Design review of the part built by this model. Coordinates are the model's own, in mm. Face numbers are marked on the shaded views. A direction names the side the tool comes from. Give positions to 0.01 mm unless a question says otherwise; leave off trailing zeros. Loops run counter-clockwise (first coordinate to the right, second up) from the corner with the lowest first, then second, coordinate; pieces in that order, holes last.
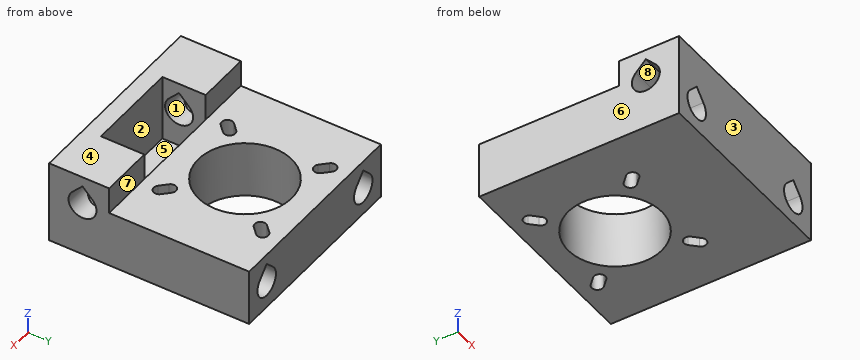
Solid Edge part; units mm, degrees
sketch "Sketch1" plane through (0, 0, 0) normal (0, 0, 1) x (1, 0, 0)
  circle A0 centre (-15.5, 15.5) radius 1.7
  circle A1 centre (15.5, 15.5) radius 1.7
  circle A2 centre (15.5, -15.5) radius 1.7
  circle A3 centre (-15.5, -15.5) radius 1.7
  line L0 (-30, -21) -> (30, -21)
  line L1 (30, -21) -> (30, 21)
  line L2 (30, 21) -> (-30, 21)
  line L3 (-30, 21) -> (-30, -21)
  circle A4 centre (0, 0) radius 14
  dimension "D1" = 30
  dimension "D2" = 30
extrude "Protrusion1" add sketch "Sketch1" along normal blind 17
sketch "Sketch2" plane through (30, 0, 8.5) normal (1, 0, 0) x (0, 1, 0)
  line L0 (-21, -8.5) -> (-39, -8.5)
  line L1 (-39, -8.5) -> (-39, 16.5)
  line L2 (-39, 16.5) -> (-21, 16.5)
  line L3 (-21, 16.5) -> (-21, -8.5)
  dimension "D1" = 21
  dimension "D2" = 39
extrude "Protrusion2" add sketch "Sketch2" against normal up to vertex (60 mm away)
sketch "Sketch3" plane through (0, 21, 8.5) normal (0, 1, 0) x (-1, 0, 0)
  line L0 (-22, 5.5461) -> (-25.0212, 2.4176)
  line L1 (-18.9788, 2.4176) -> (-22, 5.5461)
  arc A0 (-25.0212, 2.4176) -> (-18.9788, 2.4176) centre (-22, -0.5) ccw
  line L2 (22, 5.5461) -> (18.9788, 2.4176)
  line L3 (25.0212, 2.4176) -> (22, 5.5461)
  arc A1 (18.9788, 2.4176) -> (25.0212, 2.4176) centre (22, -0.5) ccw
  dimension "D1" = 22
extrude "Cutout1" cut sketch "Sketch3" against normal through all
sketch "Sketch4" plane through (30, -8, 12.5) normal (1, 0, 0) x (0, 1, 0)
  line L0 (-17.9788, 6.4176) -> (-21, 9.5461)
  line L1 (-21, 9.5461) -> (-24.0212, 6.4176)
  arc A0 (-24.0212, 6.4176) -> (-17.9788, 6.4176) centre (-21, 3.5) ccw
extrude "Cutout2" cut sketch "Sketch4" against normal through all
sketch "Sketch5" plane through (0, -30, 25) normal (0, 0, 1) x (0, -1, 0)
  line L0 (-9, -14) -> (4, -14)
  line L1 (4, -14) -> (4, 14)
  line L2 (4, 14) -> (-9, 14)
  line L3 (-9, 14) -> (-9, -14)
extrude "ExtrudedCutout_3" cut sketch "Sketch5" against normal blind 20
sketch "Sketch6" plane through (0, -9, 0) normal (0, 0, -1) x (0, 1, 0)
  line L0 (23.2979, 16.7021) -> (21.2958, 14.7)
  arc A0 (21.2958, 14.7) -> (23.7021, 12.2979) centre (22.499, 13.499) ccw
  line L1 (23.7021, 12.2979) -> (25.7021, 14.2979)
  line L2 (23.2979, 16.7021) -> (25.7021, 14.2979)
  line L3 (25.7021, -14.2979) -> (23.7, -12.2958)
  arc A1 (23.7, -12.2958) -> (21.2979, -14.7021) centre (22.499, -13.499) ccw
  line L4 (21.2979, -14.7021) -> (23.2979, -16.7021)
  arc A2 (25.7021, -14.2979) -> (23.2979, -16.7021) centre (24.5, -15.5) ccw
  line L5 (-5.2979, -16.7021) -> (-3.2958, -14.7)
  arc A3 (-3.2958, -14.7) -> (-5.7021, -12.2979) centre (-4.499, -13.499) ccw
  line L6 (-5.7021, -12.2979) -> (-7.7021, -14.2979)
  arc A4 (-5.2979, -16.7021) -> (-7.7021, -14.2979) centre (-6.5, -15.5) ccw
  line L7 (-7.7021, 14.2979) -> (-5.7, 12.2958)
  arc A5 (-5.7, 12.2958) -> (-3.2979, 14.7021) centre (-4.499, 13.499) ccw
  line L8 (-3.2979, 14.7021) -> (-5.2979, 16.7021)
  arc A6 (-7.7021, 14.2979) -> (-5.2979, 16.7021) centre (-6.5, 15.5) ccw
extrude "Cutout3" cut sketch "Sketch6" against normal through all
Q1. Draft analysis for pull direction Y (two halves, no side actions). For the marked faces 1, 2, 3 and 4, state which applies: pulls with the +Y half, pulls with the -Y half, needs draft (parallel to the pull), parting line crosses it, or undercut.
Results:
face 1: undercut
face 2: undercut
face 3: pulls with the -Y half
face 4: needs draft
Q2. Wall thickness on line 1 (Y direction, x = 0, z = 13.5); line 2 (X direction, y = -23.5, z = 8); line 3 (X direction, y = 4.5, z = 12.5): over which ranges is each line inside the solid? List them lowest first.
Results:
line 1: y = -39 to -34, -21 to -14, 14 to 21
line 2: x = -30 to -26.2, -17.8 to -14, 14 to 17.8, 26.2 to 30
line 3: x = -30 to -23.49, -20.51 to -13.26, 13.26 to 20.51, 23.49 to 30
Q3. Take a section at A-A (y = 0). Give the boundary of the cut face in (x, z), plus the area to 3 significant figures.
Results:
outline: (-30, 0) - (-14, 0) - (-14, 17) - (-30, 17) - close; (14, 0) - (30, 0) - (30, 17) - (14, 17) - close; hole (-25.02, 10.92) arc R4.2 ccw (long way) to (-18.98, 10.92) - (-22, 14.05) - close; hole (18.98, 10.92) arc R4.2 ccw (long way) to (25.02, 10.92) - (22, 14.05) - close
area: 425 mm2
Q4. Take a section at D-D (z = 8). Give the number of separate pieces and of enclosed holes in the cut face, plus the area to 3 significant figures.
Results:
separate pieces: 3
enclosed holes: 6
area: 1,540 mm2
Q5. Take a section at C-C (y = -22.5). Give the boundary of the cut face in (x, z), plus the area to 3 significant figures.
Results:
outline: (-30, 0) - (30, 0) - (30, 25) - (14, 25) - (14, 5) - (-14, 5) - (-14, 25) - (-30, 25) - close; hole (-25.02, 10.92) arc R4.2 ccw (long way) to (-18.98, 10.92) - (-22, 14.05) - close; hole (18.98, 10.92) arc R4.2 ccw (long way) to (25.02, 10.92) - (22, 14.05) - close
area: 821 mm2
Q6. Take a section at B-B (x = 15.5). Give the boundary of the cut face in (y, z), plus the area to 3 significant figures.
Results:
outline: (-39, 0) - (-17.2, 0) - (-17.2, 17) - (-21, 17) - (-21, 25) - (-39, 25) - close; (-13.1, 0) - (13.1, 0) - (13.1, 17) - (-13.1, 17) - close; (17.2, 0) - (21, 0) - (21, 17) - (17.2, 17) - close; hole (-32.02, 18.92) arc R4.2 ccw (long way) to (-25.98, 18.92) - (-29, 22.05) - close
area: 965 mm2
Q7. Tool access review of the marked faces 5, 6, 7 and 8: name each direction out of +Z, -Z, +X, -X, +Y, -Y from which nothing blocks a thin tool from reaching the whole face with its end or side.
Results:
face 5: +Z
face 6: +Z, -Z, -X, +Y, -Y
face 7: +Z, +X, -X, +Y
face 8: +X, -X
Q8. Insertion check: pin 1 (6 mm diameter, centred on x = -22.5, y = -3.5, fed in from +Z); pin 2 (4 mm diameter, centred on x = -18.5, z = 20, fed in from +Y); pin 3 (6.5 mm diameter, centred on x = 1.5, y = -24.5, fed in from +Z). Each pin has a flat end and moves straight along its axis. Give the tip position at first contact, or say it passes through.
Results:
pin 1: stops at z = 17
pin 2: stops at y = -21
pin 3: stops at z = 5
